Can you work these out from the model? Positions are in its coordinate system, mm. Face numbers are marked on the shaded views. A direction names the side the tool comes from. Round coordinates to 2 decimals unless told otherwise and drop trailing zeros. Loops run counter-clockwise (first coordinate to the right, second up) from the corner with the lowest first, then second, coordinate; pieces in that order, holes last. Notation, with made-up numbers: (72.25, 52) -> (81.25, 52) arc R17 cw to (81.25, 67) -> close; hole circle Ø1 at (-18, -31.5). An arc over 180 degrees is marked (long way). Write each question's results on one line, items separated by ' | '.
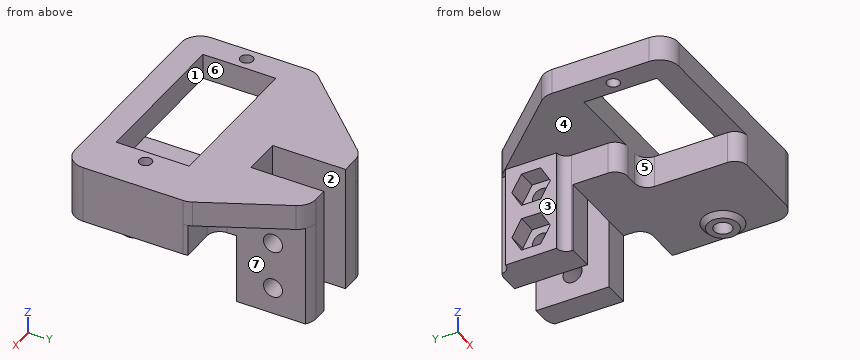
from build123d import *

# Parameters (mm, degrees)
SKETCH_1_W          = 32
SKETCH_1_H          = 19.5
SKETCH_1_R          = 1
SKETCH_1_W_2        = 24
SKETCH_1_H_2        = 11.5
SKETCH_1_W_3        = 3.5
EXTRUDE_1_DEPTH     = 4
SKETCH_4_W          = 3
SKETCH_4_H          = 3.5
EXTRUDE_3_DEPTH     = 4
FILLET_2_R          = 3
SKETCH_9_R          = 1.4
EXTRUDE_5_DEPTH     = 5
EXTRUDE_START       = 16
EXTRUDE_6_DEPTH     = 16
SKETCH_12_R         = 2.4
SKETCH_12_R_2       = 1.4
EXTRUDE_7_DEPTH     = 0.75
CHAMFER_4_SIZE      = 0.75
SKETCH_11_R         = 1.5
SKETCH_11_W         = 11
SKETCH_11_H         = 3.5
CUT_EXTRUDE_2_DEPTH = 41.720664287
FILLET_7_R          = 2
CUT_EXTRUDE_START   = -1.5
SKETCH_13_R         = 1.5
CUT_EXTRUDE_4_DEPTH = 1.5
SKETCH_15_W         = 16
SKETCH_15_H         = 8.062177826
EXTRUDE_9_DEPTH     = 1.5
FILLET_8_R          = 1.5


# Some blends are built 0.0001 mm under size
with BuildPart() as part:
    # Эскиз1 → Бобышка-Вытянуть1 (new body)
    # profile 1 of 2: a face of its own
    with BuildSketch(Plane.XY):
        Rectangle(SKETCH_1_W, SKETCH_1_H)
        with Locations((-14, 0)):
            Circle(SKETCH_1_R, mode=Mode.SUBTRACT)
        with Locations((14, 0)):
            Circle(SKETCH_1_R, mode=Mode.SUBTRACT)
        Rectangle(SKETCH_1_W_2, SKETCH_1_H_2, mode=Mode.SUBTRACT)
    # profile 2 of 2: a face of its own
    with BuildSketch(Plane.XY):
        with Locations((17.75, 0)):
            Rectangle(SKETCH_1_W_3, SKETCH_1_H)
    extrude(amount=EXTRUDE_1_DEPTH)

    # Эскиз4 → Бобышка-Вытянуть3 (add)
    with BuildSketch(Plane.XY.offset(4)):
        Polygon((-16, 9.75), (-1.9, 9.75), (-1.9, 24.75), align=None)
        Polygon((-1.9, 9.75), (2.1, 9.75), (2.1, 13.25), (2.1, 24.75), (-1.9, 24.75), align=None)
        Polygon((8.1, 13.25), (8.1, 9.75), (12.1, 9.75), (12.1, 24.75), (8.1, 24.75), align=None)
        Polygon((12.1, 24.75), (12.1, 9.75), (19.5, 9.75), align=None)
        with Locations((3.6, 11.5)):
            Rectangle(SKETCH_4_W, SKETCH_4_H)
        with Locations((6.6, 11.5)):
            Rectangle(SKETCH_4_W, SKETCH_4_H)
    extrude(amount=-EXTRUDE_3_DEPTH)

    # Скругление2
    fillet_2_edges = [part.edges().sort_by_distance(p)[0] for p in [
        (-16, 9.75, 2),
        (19.5, 9.75, 2),
        (19.5, -9.75, 2),
        (-16, -9.75, 2),
        (-1.9, 24.75, 2),
        (12.1, 24.75, 2),
    ]]
    fillet(fillet_2_edges, radius=FILLET_2_R)

    # Эскиз9 → Бобышка-Вытянуть5 (add)
    with BuildSketch(Plane(origin=(0, 0, 0), x_dir=(-1, 0, 0), z_dir=(0, 0, -1))):
        with BuildLine():
            ThreePointArc((-19.5, -6.75), (-18.621320344, -8.871320344), (-16.5, -9.75))
            Line((-16.5, -9.75), (-4, -9.75))
            Line((-4, -9.75), (-4, 5.75))
            Line((-4, 5.75), (1.9, 5.75))
            Line((1.9, 5.75), (1.9, 9.75))
            Line((1.9, 9.75), (-19.417252583, 9.75))
            ThreePointArc((-19.417252583, 9.75), (-19.479241325, 9.402567354), (-19.5, 9.050259072))
            Line((-19.5, 9.050259072), (-19.5, -6.75))
        make_face()
        with Locations(Location((-16.35, 0, 0), (0, 0, 9.875627991))):
            Circle(SKETCH_9_R, mode=Mode.SUBTRACT)
    extrude(amount=EXTRUDE_5_DEPTH)

    # Эскиз10 → Бобышка-Вытянуть6 (add)
    with BuildSketch(Plane(origin=(0, 0, 0), x_dir=(-1, 0, 0), z_dir=(0, 0, -1)).offset(EXTRUDE_START)):
        with BuildLine():
            Line((-8.1, 24.75), (-10.234794476, 24.75))
            ThreePointArc((-10.234794476, 24.75), (-11.222456407, 24.582759063), (-12.1, 24.099682607))
            Line((-12.1, 24.099682607), (-12.1, 9.75))
            Line((-12.1, 9.75), (1.9, 9.75))
            Line((1.9, 9.75), (1.9, 24.454983709))
            ThreePointArc((1.9, 24.454983709), (1.267895871, 24.675316319), (0.602670769, 24.75))
            Line((0.602670769, 24.75), (-2.1, 24.75))
            Line((-2.1, 24.75), (-2.1, 13.25))
            Line((-2.1, 13.25), (-8.1, 13.25))
            Line((-8.1, 13.25), (-8.1, 24.75))
        make_face()
    extrude(amount=-EXTRUDE_6_DEPTH)

    # Эскиз12 → Бобышка-Вытянуть7 (add)
    with BuildSketch(Plane(origin=(0, 0, -5), x_dir=(-1, 0, 0), z_dir=(0, 0, -1))):
        with Locations((-16.35, 0)):
            Circle(SKETCH_12_R)
        with Locations(Location((-16.35, 0, 0), (0, 0, 9.875627991))):
            Circle(SKETCH_12_R_2, mode=Mode.SUBTRACT)
    extrude(amount=EXTRUDE_7_DEPTH)

    # Фаска4
    chamfer_4_edges = [part.edges().sort_by_distance(p)[0] for p in [
        (18.75, 0, -5),
    ]]
    chamfer(chamfer_4_edges, length=CHAMFER_4_SIZE - 0.0001)  # a hair under: the kernel refuses the full size

    # Эскиз11 → Вырез-Вытянуть2 (cut, through all)
    with BuildSketch(Plane(origin=(12.1, 0, 0), x_dir=(0, 0, -1), z_dir=(1, 0, 0))):
        with Locations((4.25, 19)):
            Circle(SKETCH_11_R)
        with Locations((11.75, 19)):
            Circle(SKETCH_11_R)
        with Locations((10.5, 11.5)):
            Rectangle(SKETCH_11_W, SKETCH_11_H)
    extrude(amount=-CUT_EXTRUDE_2_DEPTH, mode=Mode.SUBTRACT)

    # Скругление7
    fillet_7_edges = [part.edges().sort_by_distance(p)[0] for p in [
        (4, -9.75, -2.5),
        (4, 5.75, -2.5),
        (-1.9, 5.75, -2.5),
        (12.1, 9.75, -2.5),
    ]]
    fillet(fillet_7_edges, radius=FILLET_7_R)

    # Эскиз13 → Вырез-Вытянуть4 (cut)
    # profile 1 of 2: a face of its own
    with BuildSketch(Plane.ZY.offset(1.9).offset(CUT_EXTRUDE_START)):
        Polygon((-11.75, 15.968911087), (-9.125, 17.484455543), (-9.125, 20.515544457), (-11.75, 22.031088913), (-14.375, 20.515544457), (-14.375, 17.484455543), align=None)
        with Locations(Location((-11.75, 19, 0), (0, 0, 90))):
            Circle(SKETCH_13_R, mode=Mode.SUBTRACT)
    # profile 2 of 2: a face of its own
    with BuildSketch(Plane.ZY.offset(1.9).offset(CUT_EXTRUDE_START)):
        Polygon((-1.625, 17.484455543), (-1.625, 20.515544457), (-4.25, 22.031088913), (-6.875, 20.515544457), (-6.875, 17.484455543), (-4.25, 15.968911087), align=None)
        with Locations(Location((-4.25, 19, 0), (0, 0, 90))):
            Circle(SKETCH_13_R, mode=Mode.SUBTRACT)
    extrude(amount=CUT_EXTRUDE_4_DEPTH, mode=Mode.SUBTRACT)

    # Эскиз15 → Бобышка-Вытянуть9 (add)
    with BuildSketch(Plane.ZY.offset(1.9)):
        with Locations((-8, 19)):
            Rectangle(SKETCH_15_W, SKETCH_15_H)
        Polygon((-9.125, 20.515544457), (-11.75, 22.031088913), (-14.375, 20.515544457), (-14.375, 17.484455543), (-11.75, 15.968911087), (-9.125, 17.484455543), align=None, mode=Mode.SUBTRACT)
        Polygon((-1.625, 17.484455543), (-1.625, 20.515544457), (-4.25, 22.031088913), (-6.875, 20.515544457), (-6.875, 17.484455543), (-4.25, 15.968911087), align=None, mode=Mode.SUBTRACT)
    extrude(amount=EXTRUDE_9_DEPTH)

    # Скругление8
    # the kernel refuses this fillet: 1.5 mm, written as the material it adds along each edge
    with BuildSketch(Plane(origin=(-1.9, 14.968911087, -16), x_dir=(-1, 0, 0), z_dir=(0, 0, 1))) as fillet_8_piece_1:
        with BuildLine():
            CenterArc((FILLET_8_R, FILLET_8_R), FILLET_8_R, 180, 90)
            Line((0, FILLET_8_R), (-FILLET_8_R * 0.02, FILLET_8_R))
            Line((-FILLET_8_R * 0.02, FILLET_8_R), (-FILLET_8_R * 0.02, -FILLET_8_R * 0.02))
            Line((-FILLET_8_R * 0.02, -FILLET_8_R * 0.02), (FILLET_8_R, -FILLET_8_R * 0.02))
            Line((FILLET_8_R, -FILLET_8_R * 0.02), (FILLET_8_R, 0))
        make_face()
    extrude(amount=19.75)
    with BuildSketch(Plane(origin=(-1.9, 23.031088913, 3.745170221), x_dir=(0, 1, 0), z_dir=(0, 0, -1))) as fillet_8_piece_2:
        with BuildLine():
            CenterArc((1.5, -1.498068089), FILLET_8_R, 92.908253333, 87.091746667)
            Line((0, -1.498068089), (-0.03, -1.498068089))
            Line((-0.03, -1.498068089), (-0.03, 0))
            Line((-0.03, 0), (0, 0.03))
            ThreePointArc((0, 0.03), (0.711947398, 0.03), (1.422372692, 0.029961362))
            Line((1.422372692, 0.029961362), (1.423894796, 0))
        make_face()
    extrude(amount=19.745170221)


solid = part.part
1. We'd pull the mould along X, two halves only. Please class the marked faces 4, 5, 6 and 7: pulls with the +X half, pulls with the -X half, needs draft (parallel to the pull), parting line crosses it, or undercut.
Final values:
face 4: needs draft | face 5: pulls with the -X half | face 6: undercut | face 7: pulls with the +X half
2. If we section it at D-D (z = -12.25): State how many separate pieces and enclosed holes the cut face has, then the cut area to 3 significant figures.
Final values:
separate pieces: 4 | enclosed holes: 0 | area: 69.7 mm2
3. If we section it at C-C (x = 7): List the corners of the cut face in (y, z) for me, then the cut area to 3 significant figures.
Final values:
outline: (-9.75, -5) -> (13.25, -5) -> (13.25, 4) -> (5.75, 4) -> (5.75, 0) -> (-5.75, 0) -> (-5.75, 4) -> (-9.75, 4) -> close | area: 161 mm2
4. Please list where these lines run through material, in increasing order: line 1 (Z direction, x = -2, y = 19) (3 decimals); line 2 (Y direction, x = 0.9, z = -11.75); line 3 (Y direction, x = 1.5, z = -4.25). Write a range as from..to.
Final values:
line 1: -16..-14.375, -9.125..-6.875, -1.625..4 | line 2: 13.25..17.5, 20.5..24.75 | line 3: 5.75..17.5, 20.5..24.75
5. Will these pins go through, and if not, where does the flat tip stop? pin 1 (5.5 mm diameter, centred on x = 15.5, y = 0.5, fed in from -Z); pin 2 (2.5 mm diameter, centred on y = 18, z = -10.5, fed in from -X); pin 3 (3.5 mm diameter, centred on y = 18, z = -5, fed in from +X); pin 4 (5 mm diameter, centred on x = 13, y = 20, fed in from -Z).
Final values:
pin 1: z = -5.75 | pin 2: x = -3.4 | pin 3: x = 12.1 | pin 4: z = -16
6. If we section it at B-B (x = -11.5): List the corners of the cut face in (y, z) for me, then the cut area to 3 significant figures.
Final values:
outline: (-9.75, 0) -> (-5.75, 0) -> (-5.75, 4) -> (-9.75, 4) -> close; (5.75, 0) -> (14.54, 0) -> (14.54, 4) -> (5.75, 4) -> close | area: 51.1 mm2
7. On a 3-axis mill with a long thin cutter (end or side, diameter ignored), from which of +Z, -Z, +X, -X, +Y, -Y can I reach the whole of each face in a straight line? I mean the marked faces 1, 2 and 3. Say none if no direction works.
Final values:
face 1: +Z | face 2: +Z, -Z, +Y | face 3: -Z, -X, +Y, -Y
